Autodesk Inventor part; units mm, degrees
ref_plane "YZ Plane" through (0, 0, 0) normal (1, 0, 0) x (0, 1, 0)
ref_plane "XZ Plane" through (0, 0, 0) normal (0, 1, 0) x (-1, 0, 0)
ref_plane "XY Plane" through (0, 0, 0) normal (0, 0, 1) x (1, 0, 0)
sketch "Sketch1" plane through (0, 0, 0) normal (0, 0, 1) x (1, 0, 0)
  line L0 (-21, 21) -> (21, 21)
  line L1 (21, 21) -> (21, -21)
  line L2 (21, -21) -> (-21, -21)
  line L3 (-21, -21) -> (-21, 21)
  line L4 (-21, 21) -> (21, -21) construction
  line L5 (21, 21) -> (-21, -21) construction
  point P0 (0, 0)
  dimension "d0" = 42
  dimension "d1" = 42
extrude "Extrusion1" add sketch "Sketch1" along normal mid plane 47
sketch "Sketch2" plane through (0, 0, 23.5) normal (0, 0, 1) x (1, 0, 0)
  circle A0 centre (0, 0) radius 2.5
  dimension "d4" = 5
extrude "Extrusion2" add sketch "Sketch2" along normal blind 25
sketch "Sketch3" plane through (0, 0, 23.5) normal (0, 0, 1) x (1, 0, 0)
  circle A0 centre (0, 0) radius 11
  dimension "d7" = 22
extrude "Extrusion3" add sketch "Sketch3" along normal blind 2.5
properties part number "NEMA 17 PARA TAPA PRINCIPAL"
Read the model definition and answer for the solid it produces. Units are mm, in the model's axes. A direction names the side the tool comes from. Give positions to 0.01 mm unless a question says otherwise; leave off trailing zeros. Loops run counter-clockwise (first coordinate to the right, second up) from the corner with the lowest first, then second, coordinate; pieces in that order, holes last. Notation, with made-up numbers: (52, 58) - (104, 58) arc R23 ccw to (104, 84) - close; hole circle Ø10 at (37.5, -26). An arc over 180 degrees is marked (long way). Answer as CSV lines item,"result". Start each with the question number.
1) Find section C-C (z = 31.5). Write down the section's boundary in (x, y).
2) Find section A-A (x = 0). Write down the section's boundary in (y, z), then the cut area to 3 significant figures.
3) Each of these flat-tipped pins is pushed along its axis until it touches: pin 1 Ø8 at (x, z) = (5, 29.5) entering from +Y; pin 2 Ø3 at (x, z) = (3, 33) entering from +Y; pin 3 Ø24 at (x, y) = (-4, 1) entering from +Z; pin 4 Ø4 at (y, z) = (-12, 26.5) entering from +X. Where does it stop, or does it pass through?
4) Which of the six approach directions +Z, -Z, +X, -X, +Y, -Y give full straight-line access (tool end or side, diameter ignored) to faces 1 (the face through (0, 21, 0)), 2 (the face through (-2.38, 10.74, 24.73))?
5) Find section D-D (y = -9). Write down the section's boundary in (x, z).
6) Straight lines are drawn through the part: L1, parallel to Z at x = -4, y = 12.5; L2, parallel to Z at x = 9.5, y = 4; L3, parallel to Y at x = 0.5, z = 30.5. For each, find the intervals that lie inside material, in ascending order. Write a range as from..to.
Findings below:
1,outline,"circle Ø5 at (0, 0)"
2,outline,"(-21, -23.5) - (21, -23.5) - (21, 23.5) - (11, 23.5) - (11, 26) - (2.5, 26) - (2.5, 48.5) - (-2.5, 48.5) - (-2.5, 26) - (-11, 26) - (-11, 23.5) - (-21, 23.5) - close"
2,area,"2,140 mm^2"
3,pin 1,"y = 10.56"
3,pin 2,"y = 2"
3,pin 3,"z = 48.5"
3,pin 4,"x = 4.44"
4,face 1,"+Z, -Z, +X, -X, +Y"
4,face 2,"+Z"
5,outline,"(-21, -23.5) - (21, -23.5) - (21, 23.5) - (6.32, 23.5) - (6.32, 26) - (-6.32, 26) - (-6.32, 23.5) - (-21, 23.5) - close"
6,L1,"-23.5..23.5"
6,L2,"-23.5..26"
6,L3,"-2.45..2.45"
